Autodesk Inventor part; units mm, degrees
ref_plane "YZ Plane" through (0, 0, 0) normal (1, 0, 0) x (0, 1, 0)
ref_plane "XZ Plane" through (0, 0, 0) normal (0, 1, 0) x (-1, 0, 0)
ref_plane "XY Plane" through (0, 0, 0) normal (0, 0, 1) x (1, 0, 0)
sketch "Sketch1" plane through (0, 0, 0) normal (0, 1, 0) x (-1, 0, 0)
  line L0 (9.8538, 29.2055) -> (-0.3062, 29.2055)
  line L1 (-0.3062, 29.2055) -> (-0.3062, -21.5945)
  line L2 (-0.3062, -21.5945) -> (9.8538, -21.5945)
  line L3 (9.8538, -21.5945) -> (9.8538, 29.2055)
  line L4 (4.7738, -21.5945) -> (4.7738, -16.6415)
  line L5 (4.7738, 29.2055) -> (4.7738, 24.2525)
  circle A0 centre (4.7738, 24.2525) radius 2.159
  circle A1 centre (4.7738, -16.6415) radius 2.159
  point P0 (0, 0)
  dimension "d0" = 10.16
  dimension "d1" = 50.8
  dimension "d2" = 4.953
  dimension "d3" = 4.953
  dimension "d4" = 4.318
  dimension "d5" = 4.318
extrude "Extrusion1" add sketch "Sketch1" along normal blind 7.62
fillet "Fillet1" radius 4.953 1 edges at (0.3062, 3.81, -21.5945)
fillet "Fillet2" radius 4.953 3 edges at (-9.8538, 3.81, -21.5945) (0.3062, 3.81, 29.2055) (-9.8538, 3.81, 29.2055)
properties part number "Hand4"
For this review, take the finished solid that the model builds, in its own axes (mm). Round coordinates to 2 decimals unless told otherwise and drop trailing zeros. Loops run counter-clockwise (first coordinate to the right, second up) from the corner with the lowest first, then second, coordinate; pieces in that order, holes last. Notation, with made-up numbers: (74.5, -11) - (133.5, -11) arc R33 ccw to (133.5, 18) - close; hole circle Ø2 at (83, -25.75). An arc over 180 degrees is marked (long way). Answer as CSV lines item,"result".
(1) Mouldability with a two-part tool opening along Z and no side actions: class faces 1 (the face through (-8.364, 3.863, -20.182)), 2 (the face through (-5, 0, 4)), 3 (the face through (-4.493, 3.757, 22.112)) as +Z half, -Z half, draft (parallel to the pull), parting line (faces both ways), or undercut.
Checked values:
face 1,"-Z half"
face 2,"draft"
face 3,"undercut"
(2) Consider section A-A on x = -3.25. Give the boundary of the cut face in (y, z).
Checked values:
outline,"(0, -21.39) - (7.62, -21.39) - (7.62, -18.17) - (0, -18.17) - close; (0, -15.11) - (7.62, -15.11) - (7.62, 22.72) - (0, 22.72) - close; (0, 25.78) - (7.62, 25.78) - (7.62, 29) - (0, 29) - close"
(3) Wall thickness on line 1 (Z direction, x = -6.5, y = 5.25); line 2 (Z direction, x = -5.5, y = 0.5); line 3 (X direction, y = 5, z = -15.5): over which ranges is each line inside the solid? List them lowest first.
Checked values:
line 1,"z = -21.33 to -17.94, -15.34 to 22.96, 25.55 to 28.94"
line 2,"z = -21.56 to -18.67, -14.61 to 22.22, 26.29 to 29.17"
line 3,"x = -9.85 to -6.61, -2.94 to 0.31"
(4) Consider section C-C on x = -5.5. Give the boundary of the cut face in (y, z), then the cut area to 3 significant figures.
Checked values:
outline,"(0, -21.56) - (7.62, -21.56) - (7.62, -18.67) - (0, -18.67) - close; (0, -14.61) - (7.62, -14.61) - (7.62, 22.22) - (0, 22.22) - close; (0, 26.29) - (7.62, 26.29) - (7.62, 29.17) - (0, 29.17) - close"
area,"325 mm2"
(5) Consider section B-B on y = 2.5. Give the boundary of the cut face in (x, z), then the cut area to 3 significant figures.
Checked values:
outline,"(-9.85, -16.64) arc R4.95 ccw to (-4.9, -21.59) - (-4.65, -21.59) arc R4.95 ccw to (0.31, -16.64) - (0.31, 24.25) arc R4.95 ccw to (-4.65, 29.21) - (-4.9, 29.21) arc R4.95 ccw to (-9.85, 24.25) - close; hole circle Ø4.32 at (-4.77, -16.64); hole circle Ø4.32 at (-4.77, 24.25)"
area,"466 mm2"
(6) Insertion check: P1, Ø4, axis at x = -4.77, z = -16.64, coming from the +Y side; P2, Ø3, axis at x = -8.5, y = 1, coming from the -Z side. Each pin has a flat end and moves straight along its axis. Give the tip position at first contact, or say it passes through.
Checked values:
P1,"passes through"
P2,"stops at z = -21.13"
(7) Consider section D-D on x = -1. Give the boundary of the cut face in (y, z).
Checked values:
outline,"(0, -19.99) - (7.62, -19.99) - (7.62, 27.6) - (0, 27.6) - close"
